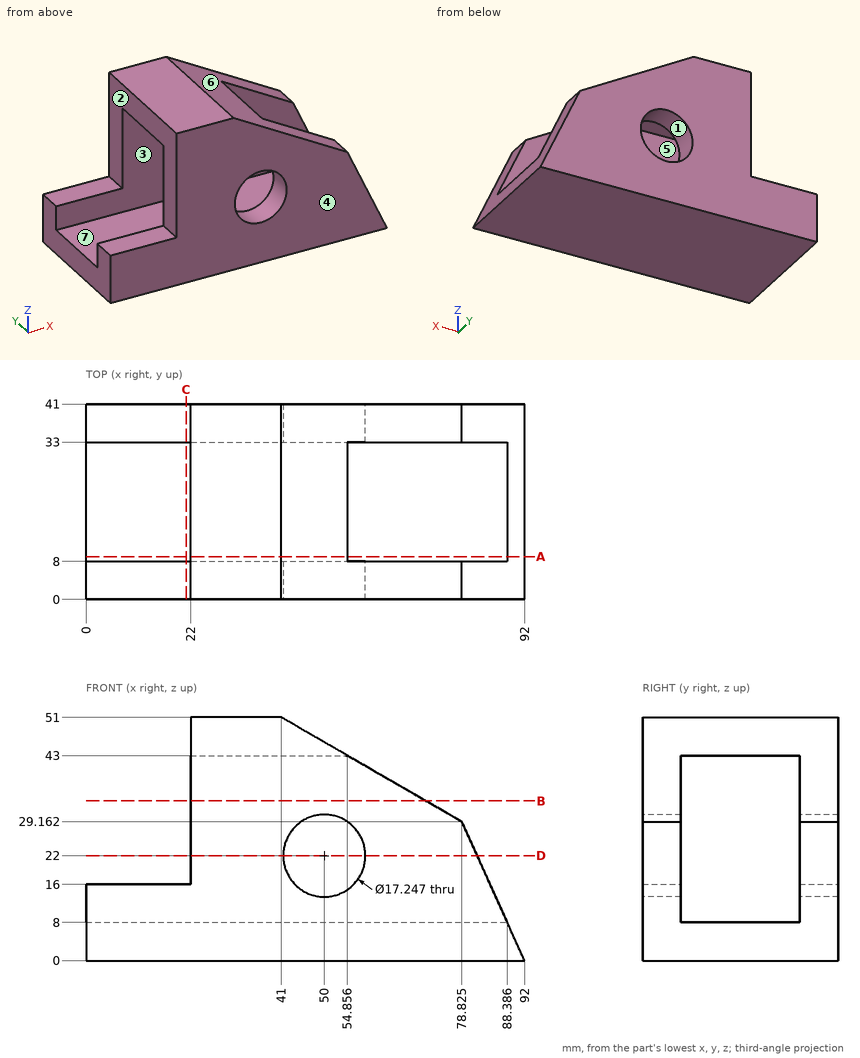
Verification items for this drawing (mm, ordinates from the low corner). A direction names the side the tool comes from. Give positions to 0.01 mm unless a question says otherwise; leave off trailing zeros. Write each loop counter-clockwise with the first axis right and the second up, starting at its lowest first coordinate (ties: lowest second). Pieces come first, ordered by that corner, then holes.
1) Section check D-D, the plane z = 22. Record the boundary of the cut face in (x, y).
2) Material ranges on L1, parallel to Y at x = 36.5, z = 38; L2, parallel to Z at x = 20.5, y = 24.5; L3, parallel to Z at x = 50, y = 2.25 (1 decimal), recorded low to high.
3) Access from +Z, -Z, +X, -X, +Y, -Y to the whole of each face (thin tool, end or side, straight path). Record for the marked faces 1, 2 and 3.
4) Gauge pin test, flat ends, axial feed: pin 1 (1 mm diameter, centred on x = 27.5, z = 28, fed in from -Y); pin 2 (8 mm diameter, centred on x = 78, z = 38, fed in from +Y); pin 3 (17.5 mm diameter, centred on y = 22, z = 39, fed in from -X); pin 4 (1.5 mm diameter, centred on y = 21.5, z = 45.5, fed in from +X) (1 decimal). Record the tip position at first contact, or that the pin passes through.
5) Section check B-B, the plane z = 33.5. Record the boundary of the cut face in (x, y), and give its area (3 significant figures).
6) Section check C-C, the plane x = 21. Record the boundary of the cut face in (y, z).
7) Section check A-A, the plane y = 9. Record the boundary of the cut face in (x, z) (1 decimal), and give its area (3 significant figures).
8) Release check for a two-part mould opening along Y. For the marked faces 4, 5, 6 and 7 record: pulls with the +Y half, pulls with the -Y half, needs draft (parallel to the pull), parting line crosses it, or undercut.
Computed:
1. outline: (22, 0) - (41.38, 0) - (41.38, 8) - (22, 8) - close; (22, 33) - (41.38, 33) - (41.38, 41) - (22, 41) - close; (58.62, 0) - (82.06, 0) - (82.06, 8) - (58.62, 8) - close; (58.62, 33) - (82.06, 33) - (82.06, 41) - (58.62, 41) - close
2. L1: y = 0 to 8, 33 to 41
2. L2: z = 0 to 8
2. L3: z = 0 to 13.4, 30.6 to 45.8
3. face 1: +Y, -Y
3. face 2: +Z, -X, +Y, -Y
3. face 3: +X, -X
4. pin 1: stops at y = 0
4. pin 2: passes through
4. pin 3: stops at x = 22
4. pin 4: stops at x = 51.8
5. outline: (22, 0) - (71.31, 0) - (71.31, 8) - (22, 8) - close; (22, 33) - (71.31, 33) - (71.31, 41) - (22, 41) - close
5. area: 789 mm2
6. outline: (0, 0) - (41, 0) - (41, 16) - (33, 16) - (33, 8) - (8, 8) - (8, 16) - (0, 16) - close
7. outline: (0, 0) - (92, 0) - (88.4, 8) - (0, 8) - close; (22, 43) - (54.9, 43) - (41, 51) - (22, 51) - close
7. area: 929 mm2
8. face 4: pulls with the -Y half
8. face 5: undercut
8. face 6: needs draft
8. face 7: undercut
